from build123d import *

# Parameters (mm, degrees)
BASE_FLANGE1_DEPTH = 100
SKETCH6_R          = 4.334335372
CUT_EXTRUDE1_DEPTH = 10


# Sheet-metal steps are written as plain solids
with BuildPart() as part:
    # Sketch1 → Base-Flange1 (new, symmetric)
    with BuildSketch(Plane.XY):
        with BuildLine():
            Line((0, 100), (0, 1))
            ThreePointArc((0, 1), (0.292893219, 0.292893219), (1, 0))
            Line((1, 0), (200, 0))
            Line((200, 0), (200, -0.7366))
            Line((200, -0.7366), (1, -0.7366))
            ThreePointArc((1, -0.7366), (-0.227961636, -0.227961636), (-0.7366, 1))
            Line((-0.7366, 1), (-0.7366, 100))
            Line((-0.7366, 100), (0, 100))
        make_face()
    extrude(amount=BASE_FLANGE1_DEPTH, both=True)

    # Sketch6 → Cut-Extrude1 (cut)
    with BuildSketch(Plane(origin=(0, 0, 0), x_dir=(1, 0, 0), z_dir=(0, 1, 0))):
        with Locations(Location((194.445286262, -82.216924087, 0), (0, 0, 270))):
            Circle(SKETCH6_R)
    extrude(amount=-CUT_EXTRUDE1_DEPTH, mode=Mode.SUBTRACT)


solid = part.part
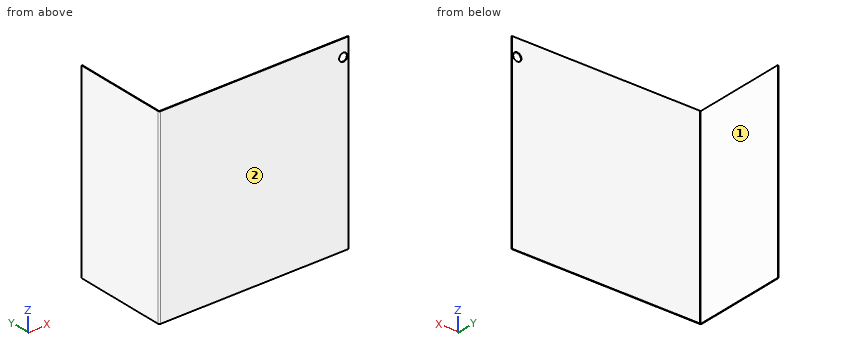
Work out the finished part from the listing and answer in its coordinate system (mm). Face numbers are marked on the shaded views. A direction names the side the tool comes from. Give positions to 0.01 mm unless a question says otherwise; leave off trailing zeros. Write each loop counter-clockwise with the first axis right and the second up, starting at its lowest first coordinate (ties: lowest second). Pieces come first, ordered by that corner, then holes. Notation, with made-up numbers: (20, 62) - (65, 62) arc R21 ccw to (65, 79) - close; hole circle Ø10 at (-21.75, 65.25). An arc over 180 degrees is marked (long way). One line per item, written item: value. Start each with the question number.
1. Given pin 1 (10 mm diameter, centred on y = 60.5, z = -72.5, fed in from +X); pin 2 (2 mm diameter, centred on x = 170.5, z = -66.5, fed in from +Y); pin 3 (8 mm diameter, centred on x = 194.45, z = 82.22, fed in from +Y), each flat-ended and moving along its own axis, determine where each tip first touches the part or whether it passes through.
2. Find section C-C (y = 60.5). Write down the section's boundary in (x, z), then the cut area to 3 significant figures.
3. Consider probe 1 along Y at (x, z) = (179, -74.5). Determine where the line is inside the solid, lowest interval first.
4. Find section A-A (z = -31). Write down the section's boundary in (x, y).
5. For the marked faces 1 and 2, determine the directions among +Z, -Z, +X, -X, +Y, -Y from which every point of the face is accessible in a straight line to the end or side of a thin tool.
6. Find section B-B (z = 80.5). Write down the section's boundary in (x, y), then the cut area to 3 significant figures.
Geometry results:
1. pin 1: x = 0
1. pin 2: y = 0
1. pin 3: through
2. outline: (-0.74, -100) - (0, -100) - (0, 100) - (-0.74, 100) - close
2. area: 147 mm2
3. probe 1: -0.74 to 0
4. outline: (-0.74, 1) arc R1.74 ccw to (1, -0.74) - (200, -0.74) - (200, 0) - (1, 0) arc R1 cw to (0, 1) - (0, 100) - (-0.74, 100) - close
5. face 1: +Z, -Z, +X, +Y
5. face 2: +Z, -Z, +X, -X, -Y
6. outline: (-0.74, 1) arc R1.74 ccw to (1, -0.74) - (190.47, -0.74) - (190.47, 0) - (1, 0) arc R1 cw to (0, 1) - (0, 100) - (-0.74, 100) - close; (198.43, -0.74) - (200, -0.74) - (200, 0) - (198.43, 0) - close
6. area: 215 mm2
